For this review, use the dimensioned drawing (mm, ordinates from the lowest corner) and the shaded views. A direction names the side the tool comes from. Round coordinates to 2 decimals unless told otherwise and drop trailing zeros. Order: outer loops, then holes, each group sorted by start corner. A loop starts at its lowest first (then second) coordinate and runs counter-clockwise, first axis right, second up. Notation, with made-up numbers: (67, 79) -> (112, 79) arc R13 cw to (112, 84) -> close; hole circle Ø4 at (19.5, 35.25). An arc over 180 degrees is marked (long way). Use a Markdown table: item, result. Add a question column.
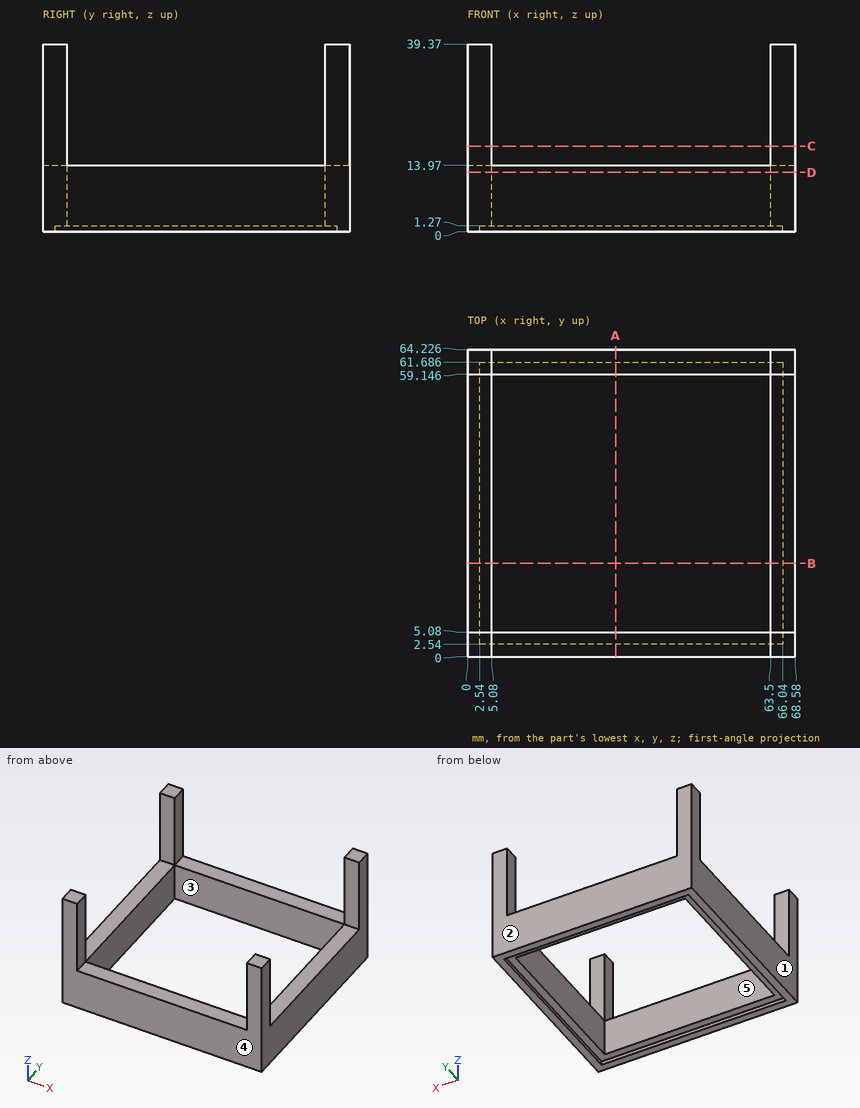
Q1. Machinability: for the marked faces 4 and 5, which of the approach directions +Z, -Z, +X, -X, +Y, -Y give a long, thin tool a straight path to every point of the face, cutting with its end or side? Answer none if there is none.
Q2. Add section D-D (z = 12.5). Write out the cut boundary in (x, y).
Q3. Add section C-C (z = 18). Write out the cut boundary in (x, y).
Q4. Mouldability with a two-part tool opening along Y and no side actions: class the marked faces 1, 2 and 3 as pulls with the +Y half, pulls with the -Y half, needs draft (parallel to the pull), parting line crosses it, or undercut.
Q5. Wall thickness on line 1 (Y direction, x = 23, z = 4); line 2 (X direction, y = 50, z = 11); line 3 (Z direction, x = 4, y = 49.5): over which ranges is each line inside the solid? List them lowest first. Write a range as [from, to].
Q6. Add section A-A (x = 31). Write out the cut boundary in (y, z).
Q7. Add section B-B (y = 19.5). Write out the cut boundary in (x, z).
Q8. Insertion check: pin 1 (10 mm diameter, centred on y = 42.5, z = 16.5, fed in from -X); pin 2 (3 mm diameter, centred on x = 29, z = 16.5, fed in from -Y); pin 3 (4 mm diameter, centred on x = 65.5, y = 30, fed in from +Z). Each pin has a flat end and moves straight along its axis. Give the tip position at first contact, or say it passes through.
Report:
| question | item | result |
|---|---|---|
| 1 | face 4 | +Z, -Z, +X, -X, -Y |
| 1 | face 5 | +Z, -Z |
| 2 | outline | (0, 0) -> (68.58, 0) -> (68.58, 64.23) -> (0, 64.23) -> close; hole (5.08, 5.08) -> (63.5, 5.08) -> (63.5, 59.15) -> (5.08, 59.15) -> close |
| 3 | outline | (0, 0) -> (5.08, 0) -> (5.08, 5.08) -> (0, 5.08) -> close; (0, 59.15) -> (5.08, 59.15) -> (5.08, 64.23) -> (0, 64.23) -> close; (63.5, 0) -> (68.58, 0) -> (68.58, 5.08) -> (63.5, 5.08) -> close; (63.5, 59.15) -> (68.58, 59.15) -> (68.58, 64.23) -> (63.5, 64.23) -> close |
| 4 | face 1 | needs draft |
| 4 | face 2 | pulls with the +Y half |
| 4 | face 3 | undercut |
| 5 | line 1 | y = [0, 5.08], [59.15, 64.23] |
| 5 | line 2 | x = [0, 5.08], [63.5, 68.58] |
| 5 | line 3 | z = [1.27, 13.97] |
| 6 | outline | (0, 0) -> (2.54, 0) -> (2.54, 1.27) -> (5.08, 1.27) -> (5.08, 13.97) -> (0, 13.97) -> close; (59.15, 1.27) -> (61.69, 1.27) -> (61.69, 0) -> (64.23, 0) -> (64.23, 13.97) -> (59.15, 13.97) -> close |
| 7 | outline | (0, 0) -> (2.54, 0) -> (2.54, 1.27) -> (5.08, 1.27) -> (5.08, 13.97) -> (0, 13.97) -> close; (63.5, 1.27) -> (66.04, 1.27) -> (66.04, 0) -> (68.58, 0) -> (68.58, 13.97) -> (63.5, 13.97) -> close |
| 8 | pin 1 | stops at x = 0 |
| 8 | pin 2 | passes through |
| 8 | pin 3 | stops at z = 13.97 |
